from build123d import *

# Parameters (mm, degrees)
SKETCH_1_W          = 15
SKETCH_1_H          = 15
SKETCH_1_W_2        = 13
SKETCH_1_H_2        = 13
EXTRUDE_1_DEPTH     = 306.44
SKETCH_2_R          = 1.45
CUT_EXTRUDE_1_DEPTH = 307.898555878
SKETCH_3_R          = 1.45
SKETCH_3_R_2        = 1.95
CUT_EXTRUDE_2_DEPTH = 307.898555878


with BuildPart() as part:
    # 草图1 → 凸台-拉伸1 (new body)
    with BuildSketch(Plane(origin=(0, 0, 0), x_dir=(0, 0, -1), z_dir=(1, 0, 0))):
        Rectangle(SKETCH_1_W, SKETCH_1_H)
        Rectangle(SKETCH_1_W_2, SKETCH_1_H_2, mode=Mode.SUBTRACT)
    extrude(amount=EXTRUDE_1_DEPTH)

    # 草图2 → 切除-拉伸1 (cut, through all)
    with BuildSketch(Plane(origin=(0, 7.5, 0), x_dir=(1, 0, 0), z_dir=(0, 1, 0))):
        with Locations(Location((20, 0, 0), (0, 0, 270))):
            Circle(SKETCH_2_R)
        with Locations(Location((12, 0, 0), (0, 0, 270))):
            Circle(SKETCH_2_R)
        with Locations(Location((37, 0, 0), (0, 0, 270))):
            Circle(SKETCH_2_R)
        with Locations(Location((53, 0, 0), (0, 0, 270))):
            Circle(SKETCH_2_R)
        with Locations(Location((156.44, 0, 0), (0, 0, 270))):
            Circle(SKETCH_2_R)
        with Locations(Location((146.44, 0, 0), (0, 0, 270))):
            Circle(SKETCH_2_R)
    extrude(amount=-CUT_EXTRUDE_1_DEPTH, mode=Mode.SUBTRACT)

    # 草图3 → 切除-拉伸2 (cut, through all)
    with BuildSketch(Plane.XY.offset(7.5)):
        with Locations((301.44, 0)):
            Circle(SKETCH_3_R)
        with Locations((291.44, 0)):
            Circle(SKETCH_3_R)
        with Locations((200, 0)):
            Circle(SKETCH_3_R_2)
        with Locations((212, 0)):
            Circle(SKETCH_3_R_2)
    extrude(amount=-CUT_EXTRUDE_2_DEPTH, mode=Mode.SUBTRACT)


solid = part.part
Geometry check sheet. Reference: the model listing, model coordinates, mm. A direction names the side the tool comes from. Round coordinates to 2 decimals unless told otherwise and drop trailing zeros. Order: outer loops, then holes, each group sorted by start corner. A loop starts at its lowest first (then second) coordinate and runs counter-clockwise, first axis right, second up. Notation, with made-up numbers: (70.5, 50) -> (128.5, 50) arc R19 cw to (128.5, 76) -> close; hole circle Ø9 at (40, 68.25). An arc over 180 degrees is marked (long way). Use one line per item in the form item = value.
1. Cross-section at B-B, the plane z = -4. Enter the section's corners in (x, y), plus the area to 3 significant figures.
Working result:
outline = (0, -7.5) -> (306.44, -7.5) -> (306.44, -6.5) -> (0, -6.5) -> close; (0, 6.5) -> (306.44, 6.5) -> (306.44, 7.5) -> (0, 7.5) -> close
area = 613 mm^2
2. Cross-section at A-A, the plane x = 136. Enter the section's corners in (y, z).
Working result:
outline = (-7.5, -7.5) -> (7.5, -7.5) -> (7.5, 7.5) -> (-7.5, 7.5) -> close; hole (-6.5, -6.5) -> (6.5, -6.5) -> (6.5, 6.5) -> (-6.5, 6.5) -> close
3. Scan lines: line 1 along Z through (x, y) = (92.5, -2); line 2 along Y through (x, z) = (200, 6.85). Record each from-to range of solid material in increasing order. Write a range as from..to.
Working result:
line_1 = -7.5..-6.5, 6.5..7.5
line_2 = -7.5..-1.95, 1.95..7.5
4. Set-up check for faces 4 (the face through (151, 6.5, 0)), 5 (the face through (0, 0, 7)): record each of +Z, -Z, +X, -X, +Y, -Y from which the full face is reachable in a straight line by a thin tool's end or side.
Working result:
face_4 = +X, -X
face_5 = +Z, -Z, -X, +Y, -Y
5. Mould release check, pull along Y, two halves, no side actions. Record for faces 1 (the face through (151, 0, -6.5)), 2 (the face through (151, 7.5, 0)), 3 (the face through (151, 0, 7.5)): pulls with the +Y half, pulls with the -Y half, needs draft (parallel to the pull), parting line crosses it, or undercut.
Working result:
face_1 = undercut
face_2 = pulls with the +Y half
face_3 = needs draft
